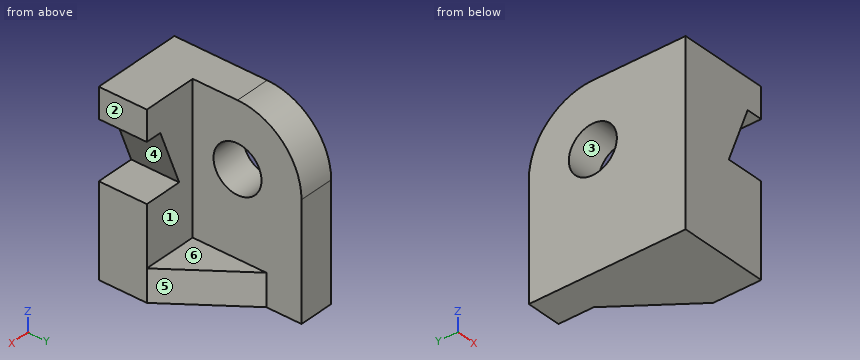
```python
from build123d import *

# Parameters (mm, degrees)
Y_KSEKLIK_EKSTR_ZYON1_DEPTH = 56
RADYUS1_R                   = 20
KES_EKSTR_ZYON1_REACH       = 65.522
IZIM2_R                     = 7.5
KES_EKSTR_ZYON2_DEPTH       = 91.210054598
KES_EKSTR_ZYON2_DEPTH_BACK  = 91.210054598
FEDER1_REACH                = 89.131
IZIM4_WALL_W                = 204.86364479
IZIM4_WALL_H                = 10


with BuildPart() as part:
    # Çizim1 → Yükseklik-Ekstrüzyon1 (new body)
    with BuildSketch(Plane.XY):
        Polygon((-62.014949412, 24.698979592), (-51.014949412, 24.698979592), (-51.014949412, -9.301020408), (-34.014949412, -9.301020408), (-34.014949412, -24.301020408), (-51.014949412, -24.301020408), (-62.014949412, -24.301020408), align=None)
    extrude(amount=Y_KSEKLIK_EKSTR_ZYON1_DEPTH)

    # Radyus1
    radyus1_edges = [part.edges().sort_by_distance(p)[0] for p in [
        (-56.514949412, 24.698979592, 56),
    ]]
    fillet(radyus1_edges, radius=RADYUS1_R)

    # Çizim2 → Kes-Ekstrüzyon1 (cut, up to next)
    with BuildSketch(Plane(origin=(-51.014949412, 0, 0), x_dir=(0, 0, -1), z_dir=(1, 0, 0)), mode=Mode.PRIVATE) as kes_ekstr_zyon1_sk1:
        with Locations(Location((-36, 4.698979592, 0), (0, 0, 90))):
            Circle(IZIM2_R)
    kes_ekstr_zyon1_tool1 = extrude(kes_ekstr_zyon1_sk1.sketch, amount=-KES_EKSTR_ZYON1_REACH, mode=Mode.PRIVATE) & part.part
    add(kes_ekstr_zyon1_tool1.solids().sort_by_distance((-51.014949, 4.69898, 36))[0], mode=Mode.SUBTRACT)

    # Çizim3 → Kes-Ekstrüzyon2 (cut, two sides: drawn at the far end of the back side and taken through both)
    with BuildSketch(Plane(origin=(0, -9.301020408, 0), x_dir=(1, 0, 0), z_dir=(0, 1, 0)).offset(-KES_EKSTR_ZYON2_DEPTH_BACK)):
        Polygon((84.737919905, -28.613266847), (-34.014949412, -28.613266847), (-46.014949412, -28.613266847), (-39.014949412, -46.613266847), (-34.014949412, -46.613266847), (84.737919905, -46.613266847), (322.24365854, -46.613266847), (322.24365854, -28.613266847), align=None)
    extrude(amount=KES_EKSTR_ZYON2_DEPTH + KES_EKSTR_ZYON2_DEPTH_BACK, mode=Mode.SUBTRACT)

    # Çizim4 wall → Feder1 (add, up to next)
    with BuildSketch(Plane(origin=(-42.514949412, 2.198979592, 0), x_dir=(-0.594391061084, 0.804176141466, 0), z_dir=(0.804176141466, 0.594391061084, 0)), mode=Mode.PRIVATE) as feder1_sk1:
        with Locations((0, 5)):
            Rectangle(IZIM4_WALL_W, IZIM4_WALL_H)
    feder1_tool1 = extrude(feder1_sk1.sketch, amount=-FEDER1_REACH, mode=Mode.PRIVATE) - part.part
    add(feder1_tool1.solids().sort_by_distance((-42.514949412, 2.198979592, 0))[0])


solid = part.part
```
Here's how the part is built. I have some questions about the finished solid (model axes, mm). Face numbers are marked on the shaded views. A direction names the side the tool comes from. Round coordinates to 2 decimals unless told otherwise and drop trailing zeros. Write each loop counter-clockwise with the first axis right and the second up, starting at its lowest first coordinate (ties: lowest second). Pieces come first, ordered by that corner, then holes.
Q1. If we mould it in two halves opening along Y, with no side actions, what happens to the marked faces 1, 2 and 3? For each: +Y half, -Y half, draft (parallel to the pull), parting line (faces both ways), or undercut.
Q2. If we section it at C-C on z = 14: Write out the boundary of the cut face in (x, y).
Q3. Please list where these lines run through material, in increasing order: probe 1 along Y at (x, z) = (-49.5, 46); probe 2 along Z at (x, y) = (-43, -6.5); probe 3 along X at (y, z) = (-7, 51.5).
Q4. Will these pins go through, and if not, where does the flat tip stop? P1, Ø24, axis at y = 4.7, z = 36, coming from the +X side; P2, Ø8, axis at x = -59, y = 10.5, coming from the +Z side.
Q5. If we section it at D-D on y = -19: Write out the boundary of the cut face in (x, z).
Q6. Which directions (+Z, -Z, +X, -X, +Y, -Y) give clear straight access to the entire face, cutting with the end or side of a thin tool? Please do the marked faces 4, 5 and 6.
Q7. If we section it at B-B on x = -58: Write out the boundary of the cut face in (y, z).
Q8. If we section it at A-A on y = 3: Write out the boundary of the cut face in (x, z).
Answer below:
1. face 1: +Y half
1. face 2: draft
1. face 3: undercut
2. outline: (-62.01, -24.3) - (-34.01, -24.3) - (-34.01, -9.3) - (-51.01, -9.3) - (-51.01, 24.7) - (-62.01, 24.7) - close
3. probe 1: y = -24.3 to -9.3
3. probe 2: z = 0 to 10
3. probe 3: x = -62.01 to -51.01
4. P1: stops at x = -51.01
4. P2: stops at z = 55.92
5. outline: (-62.01, 0) - (-34.01, 0) - (-34.01, 28.61) - (-46.01, 28.61) - (-39.01, 46.61) - (-34.01, 46.61) - (-34.01, 56) - (-62.01, 56) - close
6. face 4: +X, +Y, -Y
6. face 5: +Z, -Z, +X, +Y
6. face 6: +Z, +X, +Y
7. outline: (-24.3, 0) - (24.7, 0) - (24.7, 36) arc R20 ccw to (4.7, 56) - (-24.3, 56) - close; hole circle Ø15 at (4.7, 36)
8. outline: (-62.01, 0) - (-43.11, 0) - (-43.11, 10) - (-51.01, 10) - (-51.01, 28.69) - (-62.01, 28.69) - close; (-62.01, 43.31) - (-51.01, 43.31) - (-51.01, 56) - (-62.01, 56) - close
